The listing builds one solid part. Answer for the finished solid, in the listing's coordinates (mm). A direction names the side the tool comes from. Round coordinates to 2 decimals unless told otherwise and drop trailing zeros. Loops run counter-clockwise (first coordinate to the right, second up) from the corner with the lowest first, then second, coordinate; pieces in that order, holes last. Notation, with made-up numbers: (-38.75, 11.25) -> (-23.75, 11.25) arc R29 ccw to (-23.75, 37.25) -> close; hole circle Ø9 at (73, 87). An arc over 180 degrees is marked (long way). Write each question's results on one line, items separated by ' | '. Start each with the question number.
(1) The part is cut by section D-D (y = 143). Determine the outline of the cut face in (x, z).
(2) Determine the mould class of faces 1 (the face through (59, 3, -19)), 2 (the face through (59, 0, -20)), 3 (the face through (35.4, 102.4, -1.5)), 4 (the face through (0, 59.9, -2.7)) for opening direction Y: released by +Y, released by -Y, zero draft, split by the parting line, or undercut.
(3) Straight lines are drawn through the part: probe 1 along X at (y, z) = (134, -1); probe 2 along Y at (x, z) = (55, -1.75); probe 3 along Y at (x, z) = (78, -22.5). For each, find the intervals that lie inside material, in ascending order.
(4) Flat-ended cylindrical pins translate along their axes: pin 1 (4 mm diameter, centred on x = 35, z = -29.5, fed in from +Y); pin 2 (4.5 mm diameter, centred on x = 15, y = 44, fed in from +Z); pin 3 (1 mm diameter, centred on x = 80.5, y = 28.5, fed in from -Z); pin 4 (5 mm diameter, centred on x = 85, z = -29.5, fed in from +Y). Find the tip coordinate at first contact, or state that the pin passes through.
(5) The part is cut by section B-B (x = 55). Determine the outline of the cut face in (y, z), plus the area to 3 significant figures.
(6) The part is cut by section C-C (x = 27). Determine the outline of the cut face in (y, z).
(7) The part is cut by section A-A (z = -9.5). Determine the outline of the cut face in (x, y).
(8) For faces 5 (the face through (46, 81, -3)), 6 (the face through (56.31, 103, -1.52)), determine the directions among +Z, -Z, +X, -X, +Y, -Y from which every point of the face is accessible in a straight line to the end or side of a thin tool.
```python
from build123d import *

# Parameters (mm, degrees)
SM_BASE_FLANGE_1_DEPTH      = 120
SKETCH_6_R                  = 1.6
CUT_EXTRUDE_1_DEPTH         = 188.147001045
PATTERN_LINEAR_1_COUNT      = 2
PATTERN_LINEAR_1_PITCH      = 118
PATTERN_LINEAR_1_COUNT_DIR2 = 5
PATTERN_LINEAR_1_PITCH_DIR2 = 27
SKETCH_7_R                  = 2.1
CUT_EXTRUDE_2_DEPTH         = 188.683243791
PATTERN_LINEAR_2_COUNT      = 2
PATTERN_LINEAR_2_PITCH      = 20
PATTERN_LINEAR_2_COUNT_DIR2 = 2
PATTERN_LINEAR_2_PITCH_DIR2 = 50
M4X0_7_TAPPED_HOLE1_D       = 3.3
PATTERN_LINEAR_4_COUNT      = 3
PATTERN_LINEAR_4_PITCH      = 20
PATTERN_LINEAR_4_COUNT_DIR2 = 4
PATTERN_LINEAR_4_PITCH_DIR2 = 20
SKETCH6_W                   = 120
SKETCH6_H                   = 3
BOSS_EXTRUDE1_DEPTH         = 20
SKETCH_11_R                 = 3.02820634
SKETCH_11_R_2               = 2.816705121
EXTRUDE_1_DEPTH             = 3
M3X0_5_1_D                  = 2.5
SKETCH_13_W                 = 30
SKETCH_13_H                 = 98
CUT_EXTRUDE_3_DEPTH         = 204.039405042
FILLET_1_R                  = 5


# Sheet-metal steps are written as plain solids
with BuildPart() as part:
    # Sketch 1 → 基材-凸緣1 (new body)
    with BuildSketch(Plane(origin=(0, 0, 0), x_dir=(0, 0, -1), z_dir=(1, 0, 0))):
        with BuildLine():
            Line((35, 0), (4, 0))
            ThreePointArc((4, 0), (1.171572875, 1.171572875), (0, 4))
            Line((0, 4), (0, 140))
            Line((0, 140), (3, 140))
            Line((3, 140), (3, 4))
            ThreePointArc((3, 4), (3.292893219, 3.292893219), (4, 3))
            Line((4, 3), (35, 3))
            Line((35, 3), (35, 0))
        make_face()
    extrude(amount=SM_BASE_FLANGE_1_DEPTH)

    # 草圖6 → 除料-伸長1 (cut, through all)
    with BuildSketch(Plane(origin=(0, 0, -3), x_dir=(-1, 0, 0), z_dir=(0, 0, -1))):
        with Locations((-6, 134)):
            Circle(SKETCH_6_R)
    cut_extrude_1 = extrude(amount=-CUT_EXTRUDE_1_DEPTH, mode=Mode.SUBTRACT)

    # 直線複製排列1: Cut-Extrude 1 2 × 5, 4 skipped
    with Locations(*[(j * PATTERN_LINEAR_1_PITCH_DIR2, -i * PATTERN_LINEAR_1_PITCH, 0) for i in range(PATTERN_LINEAR_1_COUNT) for j in range(PATTERN_LINEAR_1_COUNT_DIR2) if (i, j) not in ((0, 0), (0, 1), (0, 2), (1, 1), (1, 2))]):
        add(cut_extrude_1, mode=Mode.SUBTRACT)

    # 草圖7 → 除料-伸長2 (cut, through all)
    with BuildSketch(Plane.XZ):
        with Locations(Location((35, -9.5, 0), (0, 0, 270))):
            Circle(SKETCH_7_R)
    cut_extrude_2 = extrude(amount=-CUT_EXTRUDE_2_DEPTH, mode=Mode.SUBTRACT)

    # 直線複製排列2: Cut-Extrude 2 2 × 2
    with Locations(*[(j * PATTERN_LINEAR_2_PITCH_DIR2, 0, -i * PATTERN_LINEAR_2_PITCH) for i in range(PATTERN_LINEAR_2_COUNT) for j in range(PATTERN_LINEAR_2_COUNT_DIR2) if (i, j) != (0, 0)]):
        add(cut_extrude_2, mode=Mode.SUBTRACT)

    # M4x0.7 Tapped Hole1 (through all)
    with Locations(Plane.XY):
        with Locations((15, 104)):
            m4x0_7_tapped_hole1 = Hole(M4X0_7_TAPPED_HOLE1_D / 2)

    # 直線複製排列4: M4x0.7 Tapped Hole1 3 × 4, 6 skipped
    with Locations(*[(i * PATTERN_LINEAR_4_PITCH, -j * PATTERN_LINEAR_4_PITCH_DIR2, 0) for i in range(PATTERN_LINEAR_4_COUNT) for j in range(PATTERN_LINEAR_4_COUNT_DIR2) if (i, j) not in ((0, 0), (0, 1), (0, 2), (1, 1), (1, 2), (2, 1), (2, 2))]):
        add(m4x0_7_tapped_hole1, mode=Mode.SUBTRACT)

    # Sketch6 → Boss-Extrude1 (add)
    with BuildSketch(Plane(origin=(0, 140, 0), x_dir=(1, 0, 0), z_dir=(0, 1, 0))):
        with Locations((60, 1.5)):
            Rectangle(SKETCH6_W, SKETCH6_H)
    extrude(amount=BOSS_EXTRUDE1_DEPTH)

    # 草圖11 → 填料-伸長1 (add)
    with BuildSketch(Plane.XY):
        with Locations((6, 134)):
            Circle(SKETCH_11_R)
        with Locations((6, 16)):
            Circle(SKETCH_11_R_2)
    extrude(amount=-EXTRUDE_1_DEPTH)

    # M3x0.5 螺紋孔1 (through all)
    with Locations(Plane(origin=(97, 151.5, -3), x_dir=(-1, 0, 0), z_dir=(0, 0, -1))):
        with Locations((0, 0), (90, 0), (0, -135), (90, -135)):
            Hole(M3X0_5_1_D / 2)

    # 草圖13 → 除料-伸長3 (cut, through all)
    with BuildSketch(Plane.XY):
        with Locations((105, 75)):
            Rectangle(SKETCH_13_W, SKETCH_13_H)
    extrude(amount=-CUT_EXTRUDE_3_DEPTH, mode=Mode.SUBTRACT)

    # 圓角1
    fillet_1_edges = [part.edges().sort_by_distance(p)[0] for p in [
        (120, 1.5, -35),
        (0, 1.5, -35),
        (0, 160, -1.5),
        (120, 160, -1.5),
    ]]
    fillet(fillet_1_edges, radius=FILLET_1_R)


solid = part.part
```
Checked values:
1) outline: (0, -3) -> (120, -3) -> (120, 0) -> (0, 0) -> close
2) face 1: released by +Y | face 2: released by -Y | face 3: undercut | face 4: zero draft
3) probe 1: x = 0 to 85.4, 88.6 to 112.4, 115.6 to 120 | probe 2: y = 0.69 to 42.35, 45.65 to 102.35, 105.65 to 160 | probe 3: y = 0 to 3
4) pin 1: passes through | pin 2: stops at z = 0 | pin 3: stops at z = -3 | pin 4: stops at y = 3
5) outline: (0, -35) -> (3, -35) -> (3, -4) arc R1 cw to (4, -3) -> (42.35, -3) -> (42.35, 0) -> (4, 0) arc R4 ccw to (0, -4) -> close; (45.65, -3) -> (102.35, -3) -> (102.35, 0) -> (45.65, 0) -> close; (105.65, -3) -> (160, -3) -> (160, 0) -> (105.65, 0) -> close | area: 553 mm2
6) outline: (0, -35) -> (3, -35) -> (3, -4) arc R1 cw to (4, -3) -> (160, -3) -> (160, 0) -> (4, 0) arc R4 ccw to (0, -4) -> close
7) outline: (0, 0) -> (32.9, 0) -> (32.9, 3) -> (0, 3) -> close; (37.1, 0) -> (82.9, 0) -> (82.9, 3) -> (37.1, 3) -> close; (87.1, 0) -> (120, 0) -> (120, 3) -> (87.1, 3) -> close
8) face 5: -Z, +X, -X, +Y | face 6: +Z, -Z
